from build123d import *

# Parameters (mm, degrees)
ESQUISSE2_R        = 1.5
BOSS_EXTRU_1_DEPTH = 1.5
ESQUISSE4_R        = 5
ESQUISSE4_W        = 8.5
ESQUISSE4_H        = 2.5
BOSS_EXTRU_2_DEPTH = 0.5
ESQUISSE5_W        = 5.8
ESQUISSE5_H        = 0.8
BOSS_EXTRU_3_DEPTH = 4
CONG_2_SIZE        = 2
CONG_2_SIZE_2      = 1
CONG_3_R           = 1


with BuildPart() as part:
    # Esquisse1 → Révolution1 (revolve)
    with BuildSketch(Plane.XY, mode=Mode.PRIVATE) as r_volution1_sk:
        Polygon((0, 0), (12, 0), (12, 29.5), (5.25, 29.5), (5.25, 38), (3, 38), (3, 43), (3.25, 43), (3.25, 43.25), (3, 43.25), (3, 49), (1.25, 49), (1.25, 38), (0, 38), align=None)
    revolve(r_volution1_sk.sketch.rotate(Axis((0, 0, 0), (0, -1, 0)), 180), axis=Axis((0, 0, 0), (0, -1, 0)))

    # Esquisse2 → Boss.-Extru.1 (add, symmetric)
    with BuildSketch(Plane.XY):
        with BuildLine():
            Line((0, 38), (-6, 38))
            ThreePointArc((-6, 38), (-10, 33), (-6, 28))
            Line((-6, 28), (0, 28))
            Line((0, 28), (0, 38))
        make_face()
        with Locations((-8, 33)):
            Circle(ESQUISSE2_R, mode=Mode.SUBTRACT)
    extrude(amount=BOSS_EXTRU_1_DEPTH, both=True)

    # Esquisse3 → Révolution3 (revolve)
    with BuildSketch(Plane.XY, mode=Mode.PRIVATE) as r_volution3_sk:
        Polygon((0, 36), (20, 36), (20, 36.25), (20.25, 36.25), (20.25, 36), (26, 36), (26, 34.25), (15, 34.25), (15, 33), (0, 33), align=None)
    revolve(r_volution3_sk.sketch.rotate(Axis((15, 33, 0), (1, 0, 0)), 90), axis=Axis((15, 33, 0), (1, 0, 0)))

    # Esquisse4 → Boss.-Extru.2 (add)
    with BuildSketch(Plane.XZ):
        with Locations(Location((0, 0, 0), (0, 0, 180))):
            Circle(ESQUISSE4_R)
        with Locations((0, 8)):
            Rectangle(ESQUISSE4_W, ESQUISSE4_H)
        with Locations((0, -8)):
            Rectangle(ESQUISSE4_W, ESQUISSE4_H)
    extrude(amount=BOSS_EXTRU_2_DEPTH)

    # Esquisse5 → Boss.-Extru.3 (add)
    with BuildSketch(Plane.XZ):
        with Locations((0, 8)):
            Rectangle(ESQUISSE5_W, ESQUISSE5_H)
        with Locations((0, -8)):
            Rectangle(ESQUISSE5_W, ESQUISSE5_H)
    extrude(amount=BOSS_EXTRU_3_DEPTH)

    # Congé2
    # an asymmetric fillet: 2, 1 mm, written as the material it takes off along each edge
    with BuildSketch(Plane(origin=(0, 29.5, 0), x_dir=(-1, 0, 0), z_dir=(0, 0, 1))) as cong_2_piece_1:
        with BuildLine():
            Bezier((12, CONG_2_SIZE), (12, 0), (12 - CONG_2_SIZE_2, 0), weights=[1, 0.707106781, 1])
            Line((12 - CONG_2_SIZE_2, 0), (12, 0))
            Line((12, 0), (12, CONG_2_SIZE))
        make_face()
    revolve(axis=Axis((0, 29.5, 0), (0, -1, 0)), mode=Mode.SUBTRACT)

    # Congé3
    cong_3_edges = [part.edges().sort_by_distance(p)[0] for p in [
        (12, 0, 0),
    ]]
    fillet(cong_3_edges, radius=CONG_3_R)


solid = part.part
Source: CAD feature listing. Evaluate the final solid. Frame: model axes, mm. A direction names the side the tool comes from. Coordinates: 2 decimals unless noted, no trailing zeros. Loops run counter-clockwise (first coordinate to the right, second up) from the corner with the lowest first, then second, coordinate; pieces in that order, holes last. Notation, with made-up numbers: (60, 16.25) - (110, 16.25) arc R23 ccw to (110, 52.25) - close; hole circle Ø9 at (9.25, 29.25). An arc over 180 degrees is marked (long way). One line per question, with ' | ' between items.
1) Section A-A, the plane y = 12. Return loops of the section in (x, z), then the cut area to 3 significant figures.
Report:
outline: circle Ø24 at (0, 0) | area: 452 mm²
2) Set-up query: faces 5 (the face through (23.17, 35.93, -0.65)), 6 (the face through (-2.86, 46.17, -0.9)), 7 (the face through (0, -2, 8.4)), 8 (the face through (0, -2, 7.6)), 9 (the face through (4.995, -0.246, -0.22)). Return all of +Z, -Z, +X, -X, +Y, -Y with unobstructed straight access to the full face (end or side cutting, diameter ignored); none if empty.
Report:
face 5: +X | face 6: +Y | face 7: +Z, +X, -X, -Y | face 8: +X, -X, -Y | face 9: -Y
3) First-contact query: P1, Ø4, axis at y = 29, z = 9, coming from the -X side; P2, Ø1, axis at y = 9, z = -9, coming from the +X side; P3, Ø1.8, axis at x = -1, y = -2.5, coming from the -Z side; P4, Ø3, axis at x = 0, z = -7.5, coming from the -Y side. Flat tips, straight axial feed; report the tip coordinate or a pass-through.
Report:
P1: stops at x = -9.55 | P2: stops at x = 8.47 | P3: stops at z = -8.4 | P4: stops at y = -4
4) Section B-B, the plane x = 16. Return loops of the section in (y, z).
Report:
outline: circle Ø6 at (33, 0); hole circle Ø2.5 at (33, 0)
5) Line query: line 1 along Z through (x, y) = (0, 42.25); line 2 along Y through (x, z) = (18.5, 0); line 3 along Y through (x, z) = (1, 4). Output: solid intervals per line, ascending.
Report:
line 1: z = -3 to -1.25, 1.25 to 3 | line 2: y = 30 to 31.75, 34.25 to 36 | line 3: y = -0.5 to 38
6) Pull-direction query (Z, two-part tool) for faces 1 (the face through (0, -2, -7.6)), 2 (the face through (0, -2, -8.4)), 3 (the face through (-11.446, 14.436, -3.604)), 4 (the face through (-8.325, 31.536, -0.021)); classes: released by +Z, released by -Z, zero draft, split by the parting line, or undercut.
Report:
face 1: undercut | face 2: released by -Z | face 3: split by the parting line | face 4: zero draft
